```python
from build123d import *

# Parameters (mm, degrees)
SKETCH1_W           = 11.5
SKETCH1_H           = 16.5
BOSS_EXTRUDE1_DEPTH = 0.78
SKETCH2_R           = 0.5
SKETCH2_R_2         = 1.5
CUT_EXTRUDE1_DEPTH  = 11.086297636
SKETCH2_3_R         = 0.75
SKETCH2_3_R_2       = 0.5
SKETCH2_3_R_3       = 1.75
SKETCH2_3_R_4       = 1.5
CUT_EXTRUDE2_DEPTH  = 0.05
SKETCH4_R           = 4
BOSS_EXTRUDE2_DEPTH = 15
FILLET1_R           = 1
FILLET2_R           = 0.5
SKETCH5_R           = 2
CUT_EXTRUDE3_DEPTH  = 1


with BuildPart() as part:
    # Sketch1 → Boss-Extrude1 (new body)
    with BuildSketch(Plane(origin=(0, 0, 0), x_dir=(1, 0, 0), z_dir=(0, 1, 0))):
        Rectangle(SKETCH1_W, SKETCH1_H)
    extrude(amount=BOSS_EXTRUDE1_DEPTH)

    # Sketch2 → Cut-Extrude1 (cut, through all)
    with BuildSketch(Plane(origin=(0, 0.78, 0), x_dir=(1, 0, 0), z_dir=(0, 1, 0))):
        with Locations(Location((-4.5, -7.015559496, 0), (0, 0, 270))):
            Circle(SKETCH2_R)
        with Locations(Location((-1.5, -7.015559496, 0), (0, 0, 270))):
            Circle(SKETCH2_R)
        with Locations(Location((1.5, -7.015559496, 0), (0, 0, 270))):
            Circle(SKETCH2_R)
        with Locations(Location((4.5, -7.015559496, 0), (0, 0, 270))):
            Circle(SKETCH2_R)
        with Locations(Location((-3.25, 6, 0), (0, 0, 270))):
            Circle(SKETCH2_R_2)
        with Locations(Location((3.25, 6, 0), (0, 0, 270))):
            Circle(SKETCH2_R_2)
    extrude(amount=-CUT_EXTRUDE1_DEPTH, mode=Mode.SUBTRACT)

    # Sketch2_3 → Cut-Extrude2 (cut)
    # profile 1 of 6: a face of its own
    with BuildSketch(Plane(origin=(0, 0.78, 0), x_dir=(1, 0, 0), z_dir=(0, 1, 0))):
        with Locations(Location((-4.5, -7.015559496, 0), (0, 0, 270))):
            Circle(SKETCH2_3_R)
        with Locations(Location((-4.5, -7.015559496, 0), (0, 0, 270))):
            Circle(SKETCH2_3_R_2, mode=Mode.SUBTRACT)
    # profile 2 of 6: a face of its own
    with BuildSketch(Plane(origin=(0, 0.78, 0), x_dir=(1, 0, 0), z_dir=(0, 1, 0))):
        with Locations(Location((-1.5, -7.015559496, 0), (0, 0, 270))):
            Circle(SKETCH2_3_R)
        with Locations(Location((-1.5, -7.015559496, 0), (0, 0, 270))):
            Circle(SKETCH2_3_R_2, mode=Mode.SUBTRACT)
    # profile 3 of 6: a face of its own
    with BuildSketch(Plane(origin=(0, 0.78, 0), x_dir=(1, 0, 0), z_dir=(0, 1, 0))):
        with Locations(Location((4.5, -7.015559496, 0), (0, 0, 90))):
            Circle(SKETCH2_3_R)
        with Locations(Location((4.5, -7.015559496, 0), (0, 0, 270))):
            Circle(SKETCH2_3_R_2, mode=Mode.SUBTRACT)
    # profile 4 of 6: a face of its own
    with BuildSketch(Plane(origin=(0, 0.78, 0), x_dir=(1, 0, 0), z_dir=(0, 1, 0))):
        with Locations(Location((1.5, -7.015559496, 0), (0, 0, 90))):
            Circle(SKETCH2_3_R)
        with Locations(Location((1.5, -7.015559496, 0), (0, 0, 270))):
            Circle(SKETCH2_3_R_2, mode=Mode.SUBTRACT)
    # profile 5 of 6: a face of its own
    with BuildSketch(Plane(origin=(0, 0.78, 0), x_dir=(1, 0, 0), z_dir=(0, 1, 0))):
        with Locations(Location((-3.25, 6, 0), (0, 0, 270))):
            Circle(SKETCH2_3_R_3)
        with Locations(Location((-3.25, 6, 0), (0, 0, 270))):
            Circle(SKETCH2_3_R_4, mode=Mode.SUBTRACT)
    # profile 6 of 6: a face of its own
    with BuildSketch(Plane(origin=(0, 0.78, 0), x_dir=(1, 0, 0), z_dir=(0, 1, 0))):
        with Locations(Location((3.25, 6, 0), (0, 0, 90))):
            Circle(SKETCH2_3_R_3)
        with Locations(Location((3.25, 6, 0), (0, 0, 270))):
            Circle(SKETCH2_3_R_4, mode=Mode.SUBTRACT)
    extrude(amount=-CUT_EXTRUDE2_DEPTH, mode=Mode.SUBTRACT)

    # Sketch4 → Boss-Extrude2 (add)
    with BuildSketch(Plane(origin=(0, 0.78, 0), x_dir=(1, 0, 0), z_dir=(0, 1, 0))):
        with Locations(Location((0, 0, 0), (0, 0, 90))):
            Circle(SKETCH4_R)
    extrude(amount=BOSS_EXTRUDE2_DEPTH)

    # Fillet1
    fillet1_edges = [part.edges().sort_by_distance(p)[0] for p in [
        (0, 15.78, 4),
    ]]
    fillet(fillet1_edges, radius=FILLET1_R)

    # Fillet2
    fillet2_edges = [part.edges().sort_by_distance(p)[0] for p in [
        (0, 0.78, 4),
    ]]
    fillet(fillet2_edges, radius=FILLET2_R)

    # Sketch5 → Cut-Extrude3 (cut)
    with BuildSketch(Plane(origin=(0, 15.78, 0), x_dir=(1, 0, 0), z_dir=(0, 1, 0))):
        with Locations(Location((0, 0, 0), (0, 0, 270))):
            Circle(SKETCH5_R)
    extrude(amount=-CUT_EXTRUDE3_DEPTH, mode=Mode.SUBTRACT)


solid = part.part
```
Can you work these out from the model? Positions are in its coordinate system, mm. A direction names the side the tool comes from. Give positions to 0.01 mm unless a question says otherwise; leave off trailing zeros. Loops run counter-clockwise (first coordinate to the right, second up) from the corner with the lowest first, then second, coordinate; pieces in that order, holes last. Notation, with made-up numbers: M 7,-8 L 46,-8 A13 cw 46,7 Z; hole C 53,-36.5 d9. An arc over 180 degrees is marked long. Use one line per item in the form item = value. Start each with the question number.
(1) I want a section at A-A, the plane z = -6. Write out the boundary of the cut face in (x, y).
(2) On a 3-axis mill with a long thin cutter (end or side, diameter ignored), from which of +Z, -Z, +X, -X, +Y, -Y can I reach the whole of each face in a straight line? I mean faces 4 (the cylindrical face through (1.522, 0.37, 6.516)), 5 (the flat face through (0, 14.78, 0)). Say none if no direction works.
(3) Thinking about a two-plate mould opening in X: for faces 1 (the cylindrical face through (3.905, 7.936, 0.867)), 2 (the flat face through (-3, 0.78, -4)), 3 (the cylindrical face through (5, 0.4, 7)), which applies, released by +X, released by -X, zero draft, split by the parting line, or undercut?
(4) Please list where these lines run through material, in increasing order: line 1 (X direction, y = 0.35, z = -6); line 2 (Y direction, x = 1.25, z = 5.5); line 3 (Y direction, x = 1.75, z = 2.5).
(5) I'm going to push flat-ended pins straight in: P1, Ø4, axis at x = -4, z = -5.5, coming from the +Y side; P2, Ø3, axis at y = 8, z = 2, coming from the +X side; P3, Ø0.8, axis at x = -4.5, z = 7, coming from the +Y side; P4, Ø4, axis at x = -1.5, y = 8.5, coming from the -Z side. Where does each tip first touch, or does it pass through?
(6) I want a section at B-B, the plane z = 0. Write out the boundary of the cut face in (x, y).
(7) I want a section at C-C, the plane y = 1.5. Write out the boundary of the cut face in (x, z), and give its area (3 significant figures).
Worked out:
q1.outline = M -5.75,0 L -4.75,0 L -4.75,0.73 L -5,0.73 L -5,0.78 L -5.75,0.78 Z; M -1.75,0 L 1.75,0 L 1.75,0.73 L 1.5,0.73 L 1.5,0.78 L -1.5,0.78 L -1.5,0.73 L -1.75,0.73 Z; M 4.75,0 L 5.75,0 L 5.75,0.78 L 5,0.78 L 5,0.73 L 4.75,0.73 Z
q2.face_4 = +Y, -Y
q2.face_5 = +Y
q3.face_1 = split by the parting line
q3.face_2 = zero draft
q3.face_3 = undercut
q4.line_1 = -5.75 to -4.75, -1.75 to 1.75, 4.75 to 5.75
q4.line_2 = 0 to 0.78
q4.line_3 = 0 to 15.78
q5.P1 = 0.78
q5.P2 = 3.97
q5.P3 = through
q5.P4 = -4
q6.outline = M -5.75,0 L 5.75,0 L 5.75,0.78 L 4.5,0.78 A0.5 cw 4,1.28 L 4,14.78 A1 ccw 3,15.78 L 2,15.78 L 2,14.78 L -2,14.78 L -2,15.78 L -3,15.78 A1 ccw -4,14.78 L -4,1.28 A0.5 cw -4.5,0.78 L -5.75,0.78 Z
q7.outline = C 0,0 d8
q7.area = 50.3 mm²
